Work out the finished part from the listing and answer in its coordinate system (mm). Face numbers are marked on the shaded views. A direction names the side the tool comes from. Round coordinates to 2 decimals unless told otherwise and drop trailing zeros. Order: outer loops, then holes, each group sorted by start corner. A loop starts at its lowest first (then second) coordinate and runs counter-clockwise, first axis right, second up. Notation, with made-up numbers: (2, 23) -> (51, 23) arc R34 cw to (51, 53) -> close; hole circle Ø5 at (-13, 74.25). An arc over 180 degrees is marked (long way). Use a Markdown table: item, result. Add a question column.
Item 1: A cutting plane is placed at A-A, the plane y = 0. Determine the outline of the cut face in (x, z).
Item 2: A cutting plane is placed at D-D, the plane y = 30. Determine the outline of the cut face in (x, z).
Item 3: Flat-ended cylindrical pins translate along their axes: P1, Ø22.5, axis at x = -15.5, y = -18, coming from the +Z side; P2, Ø3, axis at y = -0.5, z = 11, coming from the +X side; P3, Ø1, axis at x = 3, y = 7.5, coming from the +Z side; P4, Ø6.5, axis at y = 0, z = 15, coming from the +X side. Find the tip coordinate at first contact, or state that the pin passes through.
Item 4: A cutting plane is placed at B-B, the plane z = 13. Determine the outline of the cut face in (x, y), plus the area to 3 significant figures.
Item 5: For a pull along X with two mould halves and no side action, classify the marked faces 4, 5 and 6 as +X half, -X half, draft (parallel to the pull), parting line (faces both ways), or undercut.
Item 6: A tool of negligible diameter and unlimited length cuts with its end or side. For the marked faces 1, 2 and 3, from which of +Z, -Z, +X, -X, +Y, -Y can it reach the whole face along a straight path? Write none if from no direction.
Item 7: A cutting plane is placed at C-C, the plane x = 0. Determine the outline of the cut face in (y, z).
Item 8: Find the intervals of material crossed by L1, parallel to Z at x = -19, y = 0; L2, parallel to Y at x = -20.9, z = 15; L3, parallel to X at y = -3, z = 12, in increasing order. Write a range as [from, to].
Autodesk Fusion 360 part; units mm, degrees
sketch "Sketch1" plane through (0, 0, 0) normal (0, 0, 1) x (1, 0, 0)
  circle A0 centre (0, 0) radius 37.5
  dimension "d1" = 75
extrude "Extrude1" add sketch "Sketch1" along normal blind 5
sketch "Sketch2" plane through (0, 0, 0) normal (1, 0, 0) x (0, 1, 0)
  line L0 (-6.5, 5) -> (-6.5, 15)
  line L1 (6.5, 5) -> (6.5, 15)
  circle A0 centre (0, 15) radius 6.5
  line L2 (0, 1.75) -> (0, 22.5)
  line L3 (37.5, 5) -> (-37.5, 5)
  line L4 (-10, 5) -> (-10, 15)
  circle A1 centre (0, 15) radius 10
  line L5 (10, 5) -> (10, 15)
  line L6 (-10, 15) -> (-6.5, 15)
  line L7 (10, 15) -> (6.5, 15)
  circle A2 centre (0, 15) radius 3.5
  dimension "d4" = 13
  dimension "d5" = 10
  dimension "d6" = 20
  dimension "d14" = 7
extrude "Extrude2" add sketch "Sketch2" along normal mid plane 35 contours L0 L3 L4 A1 | L0 L3 A1 | L0 A1 L6 | L0 A0 L2 A1 | L1 L3 A1 | L1 A0 L2 A1 | L1 L3 A1 L5 | L1 A1 L7
extrude "Extrude3" add sketch "Sketch2" along normal blind 5 from surface at 17.5 contours L0 L3 L4 A1 | L0 L3 A1 | L0 A1 L6 | L0 A0 L2 A1 | L1 L3 A1 | L1 A0 L2 A1 | A0 A1 L6 L7 | A0 L2 A2 | A0 L2 A2 | L1 L3 A1 L5 | L1 A1 L7
mirror "Mirror1" about plane through (0, 0, 0) normal (1, 0, 0) of "Extrude3"
sketch "Sketch3" plane through (0, 0, 0) normal (0, 1, 0) x (1, 0, 0)
sketch "Sketch4" plane through (0, 0, 5) normal (0, 0, 1) x (-1, 0, 0)
  circle A0 centre (0, 0) radius 37.5
  line L0 (-22.5, 10) -> (22.5, 10)
  line L1 (22.5, 10) -> (22.5, -10)
  line L2 (22.5, -10) -> (-22.5, -10)
  line L3 (-22.5, -10) -> (-22.5, 10)
  circle A1 centre (0, 32.5) radius 5
  line L4 (5, 32.5) -> (5, 37.1652)
  line L5 (-5, 32.5) -> (-5, 37.1652)
  dimension "d15" = 10
extrude "Extrude4" cut sketch "Sketch4" along normal through all contours A0 A1 L4 | A0 A1 L5 | A1
equation "d7 = ( 35 / 2 ) * 1 mm"
equation "d9 = ( 35 / 2 ) * 1 mm"
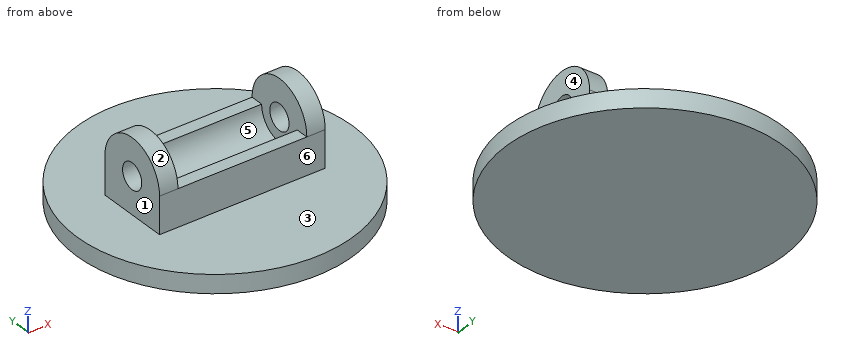
Reported:
| question | item | result |
|---|---|---|
| 1 | outline | (-37.5, 0) -> (37.5, 0) -> (37.5, 5) -> (22.5, 5) -> (22.5, 11.5) -> (17.5, 11.5) -> (17.5, 8.5) -> (-17.5, 8.5) -> (-17.5, 11.5) -> (-22.5, 11.5) -> (-22.5, 5) -> (-37.5, 5) -> close; (-22.5, 18.5) -> (-17.5, 18.5) -> (-17.5, 25) -> (-22.5, 25) -> close; (17.5, 18.5) -> (22.5, 18.5) -> (22.5, 25) -> (17.5, 25) -> close |
| 2 | outline | (-22.5, 0) -> (22.5, 0) -> (22.5, 5) -> (-22.5, 5) -> close |
| 3 | P1 | z = 22.21 |
| 3 | P2 | x = 22.5 |
| 3 | P3 | z = 15 |
| 3 | P4 | through |
| 4 | outline | (-22.5, -10) -> (22.5, -10) -> (22.5, -2.87) -> (17.5, -2.87) -> (17.5, -6.18) -> (-17.5, -6.18) -> (-17.5, -2.87) -> (-22.5, -2.87) -> close; (-22.5, 2.87) -> (-17.5, 2.87) -> (-17.5, 6.18) -> (17.5, 6.18) -> (17.5, 2.87) -> (22.5, 2.87) -> (22.5, 10) -> (-22.5, 10) -> close |
| 4 | area | 410 mm² |
| 5 | face 4 | +X half |
| 5 | face 5 | undercut |
| 5 | face 6 | draft |
| 6 | face 1 | +Z, -X, +Y, -Y |
| 6 | face 2 | +Z, +X, -X |
| 6 | face 3 | +Z |
| 7 | outline | (-37.5, 0) -> (37.5, 0) -> (37.5, 5) -> (10, 5) -> (10, 15) -> (6.5, 15) arc R6.5 cw to (-6.5, 15) -> (-10, 15) -> (-10, 5) -> (-37.5, 5) -> close |
| 8 | L1 | [0, 11.5], [18.5, 25] |
| 8 | L2 | [-10, -3.5], [3.5, 10] |
| 8 | L3 | [-22.5, -17.5], [17.5, 22.5] |
